Geometry: final body of the model. Coordinates: model frame, mm. Face numbers are marked on the shaded views. A direction names the side the tool comes from. Give positions to 0.01 mm unless a question says otherwise; leave off trailing zeros. Order: outer loops, then holes, each group sorted by start corner. A loop starts at its lowest first (then second) coordinate and runs counter-clockwise, first axis right, second up. Notation, with made-up numbers: M 62,67.5 L 104,67.5 A13 ccw 104,81.5 Z; hole C 40.5,-5.5 d10. An arc over 180 degrees is marked long. Use CSV: the item, a comma, the result in double quotes.
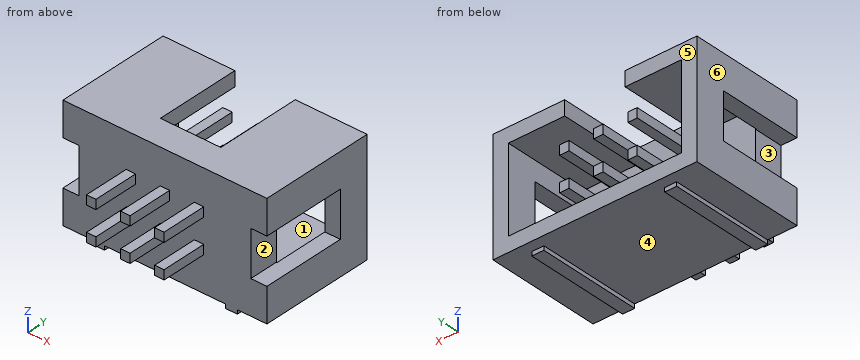
```python
from build123d import *

# Parameters (mm, degrees)
SKETCH1_W            = 15.2
SKETCH1_H            = 8.5
BOSS_EXTRUDE1_DEPTH  = 8.6
SKETCH2_W            = 12.9
SKETCH2_H            = 6.3
CUT_EXTRUDE1_DEPTH   = 6.4
SKETCH3_W            = 4.5
SKETCH3_H            = 1.1
CUT_EXTRUDE2_DEPTH   = 6.4
SKETCH4_W            = 1.2
SKETCH4_H            = 3.4
CUT_EXTRUDE3_DEPTH   = 6.3
SKETCH6_W            = 0.9
SKETCH6_H            = 0.3
BOSS_EXTRUDE2_DEPTH  = 7.8
BOSS_EXTRUDE3_START  = -8.3
SKETCH7_W            = 0.7
SKETCH7_H            = 0.7
BOSS_EXTRUDE3_DEPTH  = 11.7
LPATTERN1_COUNT      = 3
LPATTERN1_PITCH      = 2.54
LPATTERN1_COUNT_DIR2 = 2
LPATTERN1_PITCH_DIR2 = 2.54


with BuildPart() as part:
    # Sketch1 → Boss-Extrude1 (new body)
    with BuildSketch(Plane(origin=(0, 0, 0), x_dir=(1, 0, 0), z_dir=(0, 1, 0))):
        Rectangle(SKETCH1_W, SKETCH1_H)
    extrude(amount=BOSS_EXTRUDE1_DEPTH)

    # Sketch2 → Cut-Extrude1 (cut)
    with BuildSketch(Plane(origin=(0, 8.6, 0), x_dir=(1, 0, 0), z_dir=(0, 1, 0))):
        Rectangle(SKETCH2_W, SKETCH2_H)
    extrude(amount=-CUT_EXTRUDE1_DEPTH, mode=Mode.SUBTRACT)

    # Sketch3 → Cut-Extrude2 (cut)
    with BuildSketch(Plane(origin=(0, 8.6, 0), x_dir=(1, 0, 0), z_dir=(0, 1, 0))):
        with Locations((0, -3.7)):
            Rectangle(SKETCH3_W, SKETCH3_H)
    extrude(amount=-CUT_EXTRUDE2_DEPTH, mode=Mode.SUBTRACT)

    # Sketch4 → Cut-Extrude3 (cut)
    with BuildSketch(Plane.XZ):
        with Locations((7, 0)):
            Rectangle(SKETCH4_W, SKETCH4_H)
    cut_extrude3 = extrude(amount=-CUT_EXTRUDE3_DEPTH, mode=Mode.SUBTRACT)

    # Sketch6 → Boss-Extrude2 (add)
    with BuildSketch(Plane.XZ):
        with Locations((4.95, -4.4)):
            Rectangle(SKETCH6_W, SKETCH6_H)
    boss_extrude2 = extrude(amount=-BOSS_EXTRUDE2_DEPTH)

    # Mirror1: Cut-Extrude3, Boss-Extrude2 across plane
    add(cut_extrude3.mirror(Plane(origin=(0, 0, 0), x_dir=(0, 0, 1), z_dir=(1, 0, 0))), mode=Mode.SUBTRACT)
    add(boss_extrude2.mirror(Plane(origin=(0, 0, 0), x_dir=(0, 0, 1), z_dir=(1, 0, 0))))

    # Sketch7 → Boss-Extrude3 (add)
    with BuildSketch(Plane.XZ.offset(BOSS_EXTRUDE3_START)):
        with Locations((-2.54, -1.27)):
            Rectangle(SKETCH7_W, SKETCH7_H)
    boss_extrude3 = extrude(amount=BOSS_EXTRUDE3_DEPTH)

    # LPattern1: Boss-Extrude3 3 × 2
    with Locations(*[(i * LPATTERN1_PITCH, 0, j * LPATTERN1_PITCH_DIR2) for i in range(LPATTERN1_COUNT) for j in range(LPATTERN1_COUNT_DIR2) if (i, j) != (0, 0)]):
        add(boss_extrude3)


solid = part.part
```
1. Section D-D, the plane z = 3.75. Return the cut outline in (x, y).
Answer:
outline,"M -7.6,0 L 7.6,0 L 7.6,8.6 L 2.25,8.6 L 2.25,2.2 L -2.25,2.2 L -2.25,8.6 L -7.6,8.6 Z"
2. Section B-B, the plane x = -3.5. Return the cut outline in (y, z).
Answer:
outline,"M 0,-4.25 L 8.6,-4.25 L 8.6,-3.15 L 2.2,-3.15 L 2.2,3.15 L 8.6,3.15 L 8.6,4.25 L 0,4.25 Z"
3. Reachability of the marked faces 1, 2 and 3 from +Z, -Z, +X, -X, +Y, -Y: full face, straight path, thin tool, end or side. Return the list, or none.
Answer:
face 1,"+Y"
face 2,"+X, +Y, -Y"
face 3,"-X, +Y, -Y"
4. Pull-direction query (X, two-part tool) for the marked faces 4, 5 and 6; classes: +X half, -X half, draft (parallel to the pull), parting line (faces both ways), or undercut.
Answer:
face 4,"undercut"
face 5,"draft"
face 6,"-X half"
5. Line query: line 1 (X direction, y = -2, z = -1.25); line 2 (X direction, y = 6.75, z = 2.25); line 3 (Z direction, x = 4.25, y = 6.75). Output: solid intervals per line, ascending.
Answer:
line 1,"-2.89 to -2.19, -0.35 to 0.35, 2.19 to 2.89"
line 2,"-7.6 to -6.45, 6.45 to 7.6"
line 3,"-4.25 to -3.15, 3.15 to 4.25"
6. Section A-A, the plane y = 7.5. Give the number of separate pieces and of enclosed holes in the cut face, plus the area to 3 significant figures.
Answer:
separate pieces,"7"
enclosed holes,"0"
area,"46.5 mm2"
7. Pin query (flat end, axial travel): pin 1 Ø0.8 at (y, z) = (-2.5, -1.5) entering from +X; pin 2 Ø0.8 at (x, z) = (2.5, -1) entering from +Y. Return the tip coordinate at first contact, or that it passes through.
Answer:
pin 1,"x = 2.89"
pin 2,"y = 8.3"
